from build123d import *

# Parameters (mm, degrees)
CROQUIS1_R                 = 12.7
CROQUIS1_R_2               = 10.5
SALIENTE_EXTRUIR1_DEPTH    = 200
CROQUIS2_R                 = 1.5
CORTAR_EXTRUIR1_DEPTH      = 13.7
CORTAR_EXTRUIR1_DEPTH_BACK = 13.7


with BuildPart() as part:
    # Croquis1 → Saliente-Extruir1 (new body)
    with BuildSketch(Plane(origin=(0, 0, 0), x_dir=(1, 0, 0), z_dir=(0, 1, 0))):
        Circle(CROQUIS1_R)
        Circle(CROQUIS1_R_2, mode=Mode.SUBTRACT)
    extrude(amount=SALIENTE_EXTRUIR1_DEPTH)

    # Croquis2 → Cortar-Extruir1 (cut, two sides)
    with BuildSketch(Plane.XY) as cortar_extruir1_sk:
        with Locations((0, 190)):
            Circle(CROQUIS2_R)
        with Locations((0, 10)):
            Circle(CROQUIS2_R)
    extrude(amount=CORTAR_EXTRUIR1_DEPTH, mode=Mode.SUBTRACT)
    extrude(cortar_extruir1_sk.sketch, amount=-CORTAR_EXTRUIR1_DEPTH_BACK, mode=Mode.SUBTRACT)


solid = part.part
Geometry: final body of the model. Coordinates: model frame, mm. Coordinates: 2 decimals unless noted, no trailing zeros. Order: outer loops, then holes, each group sorted by start corner. A loop starts at its lowest first (then second) coordinate and runs counter-clockwise, first axis right, second up.
(1) Section query A-A (x = 5.75). Return the cut outline in (y, z).
(2) Section query C-C (y = 29). Return the cut outline in (x, z), plus the area to 3 significant figures.
(3) First-contact query: pin 1 (3 mm diameter, centred on y = 27, z = 9, fed in from -X); pin 2 (4 mm diameter, centred on x = 5, y = 43.5, fed in from -Z); pin 3 (6 mm diameter, centred on x = 7, y = 48, fed in from +Z); pin 4 (4 mm diameter, centred on x = -3.5, z = 8, fed in from +Y). Flat tips, straight axial feed; report the tip coordinate or a pass-through.
(4) Section query B-B (z = 6). Return the cut outline in (x, y).
(5) Draft query along X for faces 1 (the face through (-8, 0, -8)), 2 (the face through (-2.75, 98.6, 12.4)), 3 (the face through (4.845, 98.6, 9.315)). Return one class per face: pulls with the +X half, pulls with the -X half, needs draft (parallel to the pull), parting line crosses it, or undercut.
(6) Material intervals for probe 1 along Y at (x, z) = (0, 11.45); probe 2 along Z at (x, y) = (-0.25, 146.5), sorted ascending.
Solution:
1. outline: (0, -11.32) - (200, -11.32) - (200, -8.79) - (0, -8.79) - close; (0, 8.79) - (200, 8.79) - (200, 11.32) - (0, 11.32) - close
2. outline: circle Ø25.4 at (0, 0); hole circle Ø21 at (0, 0)
2. area: 160 mm2
3. pin 1: stops at x = -10.25
3. pin 2: stops at z = -12.34
3. pin 3: stops at z = 12.05
3. pin 4: stops at y = 200
4. outline: (-11.19, 0) - (-8.62, 0) - (-8.62, 200) - (-11.19, 200) - close; (8.62, 0) - (11.19, 0) - (11.19, 200) - (8.62, 200) - close
5. face 1: needs draft
5. face 2: parting line crosses it
5. face 3: undercut
6. probe 1: y = 0 to 8.5, 11.5 to 188.5, 191.5 to 200
6. probe 2: z = -12.7 to -10.5, 10.5 to 12.7
